```python
from build123d import *

# Parameters (mm, degrees)
SKETCH1_W                        = 56.14
SKETCH1_H                        = 20
BOSS_EXTRUDE1_DEPTH              = 2.49
M3_CLEARANCE_HOLE1_D             = 3.4
M3_CLEARANCE_HOLE1_DEPTH         = 19
M3_CLEARANCE_HOLE1_TIP           = 1.021463052
SKETCH4_W                        = 41.03
SKETCH4_H                        = 20
BOSS_EXTRUDE2_DEPTH              = 8.58
SKETCH5_R                        = 2.98
SKETCH5_R_2                      = 0.928997072
BOSS_EXTRUDE3_DEPTH              = 3.75
SKETCH6_W                        = 8
SKETCH6_H                        = 20
BOSS_EXTRUDE4_DEPTH              = 20
BOSS_EXTRUDE4_2_DEPTH            = 20
SKETCH7_W                        = 41.03
SKETCH7_H                        = 20
BOSS_EXTRUDE5_DEPTH              = 20
SKETCH8_W                        = 56.14
SKETCH8_H                        = 20
BOSS_EXTRUDE6_DEPTH              = 2.46
SKETCH12_W                       = 1.7
SKETCH12_H                       = 24.95
M3_CLEARANCE_HOLE2_AT_2_COUNT    = 2
M3_CLEARANCE_HOLE2_AT_2_PITCH    = 10
M3_CLEARANCE_HOLE2_AT_3_COUNT    = 2
M3_CLEARANCE_HOLE2_AT_3_PITCH    = 50
M3_CLEARANCE_HOLE2_AT_4_COUNT    = 2
M3_CLEARANCE_HOLE2_AT_4_PITCH    = 50.990195136
SKETCH13_W                       = 41.03
SKETCH13_H                       = 20
BOSS_EXTRUDE7_DEPTH              = 39
SKETCH14_R                       = 4
SKETCH14_R_2                     = 1.25
BOSS_EXTRUDE8_DEPTH              = 5.37
SKETCH16_W                       = 0.8
SKETCH16_H                       = 20.00005
TAP_DRILL_FOR_M2_TAP1_AT_2_COUNT = 2
TAP_DRILL_FOR_M2_TAP1_AT_2_PITCH = 25.495097568
TAP_DRILL_FOR_M2_TAP1_AT_3_COUNT = 2
TAP_DRILL_FOR_M2_TAP1_AT_3_PITCH = 10
TAP_DRILL_FOR_M2_TAP1_AT_4_COUNT = 2
TAP_DRILL_FOR_M2_TAP1_AT_4_PITCH = 50
TAP_DRILL_FOR_M2_TAP1_AT_5_COUNT = 2
TAP_DRILL_FOR_M2_TAP1_AT_5_PITCH = 50.990195136
CHAMFER1_SIZE                    = 2
SKETCH19_R                       = 6.18
SKETCH19_R_2                     = 4
BOSS_EXTRUDE10_DEPTH             = 2.12
SKETCH21_W                       = 8
SKETCH21_H                       = 7
CUT_EXTRUDE1_DEPTH               = 28
SKETCH22_W                       = 20
SKETCH22_H                       = 20
CUT_EXTRUDE2_DEPTH               = 8.235
SKETCH23_W                       = 20
SKETCH23_H                       = 20
CUT_EXTRUDE3_DEPTH               = 8.235


with BuildPart() as part:
    # Sketch1 → Boss-Extrude1 (new body)
    with BuildSketch(Plane.XY):
        Rectangle(SKETCH1_W, SKETCH1_H)
    extrude(amount=BOSS_EXTRUDE1_DEPTH)

    # M3 Clearance Hole1
    with Locations(Plane.XY.offset(2.49)):
        with Locations((25, 5), (0, 0), (-25, 5), (-25, -5), (25, -5)):
            Hole(M3_CLEARANCE_HOLE1_D / 2, depth=M3_CLEARANCE_HOLE1_DEPTH)
            with Locations((0, 0, -(M3_CLEARANCE_HOLE1_DEPTH + M3_CLEARANCE_HOLE1_TIP / 2))):  # 118° drill point
                Cone(0, M3_CLEARANCE_HOLE1_D / 2, M3_CLEARANCE_HOLE1_TIP, mode=Mode.SUBTRACT)

    # Sketch4 → Boss-Extrude2 (add)
    with BuildSketch(Plane.XY.offset(2.49)):
        Rectangle(SKETCH4_W, SKETCH4_H)
    extrude(amount=BOSS_EXTRUDE2_DEPTH)

    # Sketch5 → Boss-Extrude3 (add)
    with BuildSketch(Plane.XY.offset(11.07)):
        with Locations((8.73, 0)):
            Circle(SKETCH5_R)
        with Locations((8.73, 0)):
            Circle(SKETCH5_R_2, mode=Mode.SUBTRACT)
    extrude(amount=BOSS_EXTRUDE3_DEPTH)

    # Sketch7 → Boss-Extrude5 (add)
    with BuildSketch(Plane(origin=(0, 0, 0), x_dir=(-1, 0, 0), z_dir=(0, 0, -1))):
        Rectangle(SKETCH7_W, SKETCH7_H)
    extrude(amount=BOSS_EXTRUDE5_DEPTH)

    # Sketch8 → Boss-Extrude6 (add)
    with BuildSketch(Plane(origin=(0, 0, -20), x_dir=(-1, 0, 0), z_dir=(0, 0, -1))):
        Rectangle(SKETCH8_W, SKETCH8_H)
    extrude(amount=BOSS_EXTRUDE6_DEPTH)


with BuildPart() as body_2:
    # Sketch6 → Boss-Extrude4 (new body)
    with BuildSketch(Plane(origin=(0, 0, 0), x_dir=(-1, 0, 0), z_dir=(0, 0, -1))):
        with Locations((-24.75, 0)):
            Rectangle(SKETCH6_W, SKETCH6_H)
    extrude(amount=BOSS_EXTRUDE4_DEPTH)


with BuildPart() as body_3:
    # Sketch6 → Boss-Extrude4 2 (new body)
    with BuildSketch(Plane(origin=(0, 0, 0), x_dir=(-1, 0, 0), z_dir=(0, 0, -1))):
        with Locations((24.75, 0)):
            Rectangle(SKETCH6_W, SKETCH6_H)
    extrude(amount=BOSS_EXTRUDE4_2_DEPTH)


with BuildPart() as m3_clearance_hole2_tool:
    # Sketch12 → M3 Clearance Hole2 (revolve)
    with BuildSketch(Plane(origin=(25, 5, 2.49), x_dir=(0, -1, 0), z_dir=(1, 0, 0))):
        with Locations((0.85, 12.475)):
            Rectangle(SKETCH12_W, SKETCH12_H)
    m3_clearance_hole2 = revolve(axis=Axis((25, 5, 8.84), (0, 0, -1)))


with BuildPart() as part_1:
    add(part.part)

    # M3 Clearance Hole2: cut by m3_clearance_hole2_tool
    add(m3_clearance_hole2_tool.part, mode=Mode.SUBTRACT)


with BuildPart() as body_2_1:
    add(body_2.part)

    # M3 Clearance Hole2: cut by m3_clearance_hole2_tool
    add(m3_clearance_hole2_tool.part, mode=Mode.SUBTRACT)


with BuildPart() as m3_clearance_hole2_at_2_tool:
    # M3 Clearance Hole2 at 2: M3 Clearance Hole2 ×2
    with Locations(*[(0, -i * M3_CLEARANCE_HOLE2_AT_2_PITCH, 0) for i in range(1, M3_CLEARANCE_HOLE2_AT_2_COUNT)]):
        add(m3_clearance_hole2)


with BuildPart() as part_2:
    add(part_1.part)

    # M3 Clearance Hole2 at 2: cut by m3_clearance_hole2_at_2_tool
    add(m3_clearance_hole2_at_2_tool.part, mode=Mode.SUBTRACT)


with BuildPart() as body_2_2:
    add(body_2_1.part)

    # M3 Clearance Hole2 at 2: cut by m3_clearance_hole2_at_2_tool
    add(m3_clearance_hole2_at_2_tool.part, mode=Mode.SUBTRACT)


with BuildPart() as m3_clearance_hole2_at_3_tool:
    # M3 Clearance Hole2 at 3: M3 Clearance Hole2 ×2
    with Locations(*[(-i * M3_CLEARANCE_HOLE2_AT_3_PITCH, 0, 0) for i in range(1, M3_CLEARANCE_HOLE2_AT_3_COUNT)]):
        add(m3_clearance_hole2)


with BuildPart() as part_3:
    add(part_2.part)

    # M3 Clearance Hole2 at 3: cut by m3_clearance_hole2_at_3_tool
    add(m3_clearance_hole2_at_3_tool.part, mode=Mode.SUBTRACT)


with BuildPart() as body_3_1:
    add(body_3.part)

    # M3 Clearance Hole2 at 3: cut by m3_clearance_hole2_at_3_tool
    add(m3_clearance_hole2_at_3_tool.part, mode=Mode.SUBTRACT)


with BuildPart() as m3_clearance_hole2_at_4_tool:
    # M3 Clearance Hole2 at 4: M3 Clearance Hole2 ×2
    with Locations(*[Vector(-0.9805806756909201, -0.19611613513818418, 0) * (i * M3_CLEARANCE_HOLE2_AT_4_PITCH) for i in range(1, M3_CLEARANCE_HOLE2_AT_4_COUNT)]):
        add(m3_clearance_hole2)


with BuildPart() as part_4:
    add(part_3.part)

    # M3 Clearance Hole2 at 4: cut by m3_clearance_hole2_at_4_tool
    add(m3_clearance_hole2_at_4_tool.part, mode=Mode.SUBTRACT)

    # Sketch13 → Boss-Extrude7 (add)
    with BuildSketch(Plane.XY.offset(11.07)):
        Rectangle(SKETCH13_W, SKETCH13_H)
    extrude(amount=-BOSS_EXTRUDE7_DEPTH)

    # Sketch14 → Boss-Extrude8 (add)
    with BuildSketch(Plane(origin=(0, 0, -27.93), x_dir=(-1, 0, 0), z_dir=(0, 0, -1))):
        with Locations(Location((-8.73, 0, 0), (0, 0, 180))):
            Circle(SKETCH14_R)
        with Locations(Location((-8.73, 0, 0), (0, 0, 180))):
            Circle(SKETCH14_R_2, mode=Mode.SUBTRACT)
    extrude(amount=BOSS_EXTRUDE8_DEPTH)


with BuildPart() as body_3_2:
    add(body_3_1.part)

    # M3 Clearance Hole2 at 4: cut by m3_clearance_hole2_at_4_tool
    add(m3_clearance_hole2_at_4_tool.part, mode=Mode.SUBTRACT)

    # Sketch16 → Tap Drill for M2 Tap1 (revolve, cut)
    with BuildSketch(Plane(origin=(-25, -10, -5), x_dir=(0, 0, -1), z_dir=(1, 0, 0))):
        with Locations((0.4, 10.000025)):
            Rectangle(SKETCH16_W, SKETCH16_H)
    tap_drill_for_m2_tap1 = revolve(axis=Axis((-25, -16.35, -5), (0, 1, 0)), mode=Mode.SUBTRACT)

    # Tap Drill for M2 Tap1 at 3: Tap Drill for M2 Tap1 ×2
    with Locations(*[(0, 0, -i * TAP_DRILL_FOR_M2_TAP1_AT_3_PITCH) for i in range(1, TAP_DRILL_FOR_M2_TAP1_AT_3_COUNT)]):
        add(tap_drill_for_m2_tap1, mode=Mode.SUBTRACT)


with BuildPart() as part_5:
    add(part_4.part)

    # Tap Drill for M2 Tap1 at 2: Tap Drill for M2 Tap1 ×2
    with Locations(*[Vector(0.9805806756909201, 0, -0.1961161351381842) * (i * TAP_DRILL_FOR_M2_TAP1_AT_2_PITCH) for i in range(1, TAP_DRILL_FOR_M2_TAP1_AT_2_COUNT)]):
        add(tap_drill_for_m2_tap1, mode=Mode.SUBTRACT)

    # Chamfer1
    chamfer1_edges = [part_5.edges().sort_by_distance(p)[0] for p in [
        (-20.515, 0, 11.07),
        (20.515, 0, 11.07),
    ]]
    chamfer(chamfer1_edges, length=CHAMFER1_SIZE)

    # Sketch19 → Boss-Extrude10 (add)
    with BuildSketch(Plane(origin=(0, 0, -27.93), x_dir=(-1, 0, 0), z_dir=(0, 0, -1))):
        with Locations(Location((-8.73, 0, 0), (0, 0, 180))):
            Circle(SKETCH19_R)
        with Locations(Location((-8.73, 0, 0), (0, 0, 180))):
            Circle(SKETCH19_R_2, mode=Mode.SUBTRACT)
    extrude(amount=BOSS_EXTRUDE10_DEPTH)


with BuildPart() as body_2_3:
    add(body_2_2.part)

    # Tap Drill for M2 Tap1 at 4: Tap Drill for M2 Tap1 ×2
    with Locations(*[(i * TAP_DRILL_FOR_M2_TAP1_AT_4_PITCH, 0, 0) for i in range(1, TAP_DRILL_FOR_M2_TAP1_AT_4_COUNT)]):
        add(tap_drill_for_m2_tap1, mode=Mode.SUBTRACT)

    # Tap Drill for M2 Tap1 at 5: Tap Drill for M2 Tap1 ×2
    with Locations(*[Vector(0.9805806756909202, 0, -0.19611613513818407) * (i * TAP_DRILL_FOR_M2_TAP1_AT_5_PITCH) for i in range(1, TAP_DRILL_FOR_M2_TAP1_AT_5_COUNT)]):
        add(tap_drill_for_m2_tap1, mode=Mode.SUBTRACT)


with BuildPart() as cut_extrude1_tool:
    # Sketch21 → Cut-Extrude1 (new body)
    with BuildSketch(Plane(origin=(0, 10, 0), x_dir=(1, 0, 0), z_dir=(0, 1, 0))):
        with Locations((-24.75, 10)):
            Rectangle(SKETCH21_W, SKETCH21_H)
        with Locations((24.75, 10)):
            Rectangle(SKETCH21_W, SKETCH21_H)
    extrude(amount=-CUT_EXTRUDE1_DEPTH)


with BuildPart() as body_2_4:
    add(body_2_3.part)

    # Cut-Extrude1: cut by cut_extrude1_tool
    add(cut_extrude1_tool.part, mode=Mode.SUBTRACT)


with BuildPart() as body_3_3:
    add(body_3_2.part)

    # Cut-Extrude1: cut by cut_extrude1_tool
    add(cut_extrude1_tool.part, mode=Mode.SUBTRACT)


with BuildPart() as cut_extrude1_piece_1:
    # of the separate pieces the step leaves, piece 1, a body of its own (cut_extrude1_pieces)
    add(body_2_4.part.solids().sort_by_distance((20.75, 10, 0))[0])


with BuildPart() as cut_extrude1_piece_2:
    # of the separate pieces the step leaves, piece 2, a body of its own (cut_extrude1_pieces)
    add(body_2_4.part.solids().sort_by_distance((20.75, 10, -13.5))[0])


with BuildPart() as cut_extrude1_piece_1_of_body_3:
    # of the separate pieces the step leaves, piece 1, a body of its own (cut_extrude1_pieces_of_body_3)
    add(body_3_3.part.solids().sort_by_distance((-28.75, 10, 0))[0])


with BuildPart() as cut_extrude1_piece_2_of_body_3:
    # of the separate pieces the step leaves, piece 2, a body of its own (cut_extrude1_pieces_of_body_3)
    add(body_3_3.part.solids().sort_by_distance((-28.75, 10, -13.5))[0])


with BuildPart() as cut_extrude2_tool:
    # Sketch22 → Cut-Extrude2 (new body)
    with BuildSketch(Plane.ZY.offset(28.75)):
        with Locations((-10, 0)):
            Rectangle(SKETCH22_W, SKETCH22_H)
    extrude(amount=-CUT_EXTRUDE2_DEPTH)


with BuildPart() as cut_extrude1_piece_1_of_body_3_1:
    add(cut_extrude1_piece_1_of_body_3.part)

    # Cut-Extrude2: cut by cut_extrude2_tool
    add(cut_extrude2_tool.part, mode=Mode.SUBTRACT)


with BuildPart() as cut_extrude1_piece_2_of_body_3_1:
    add(cut_extrude1_piece_2_of_body_3.part)

    # Cut-Extrude2: cut by cut_extrude2_tool
    add(cut_extrude2_tool.part, mode=Mode.SUBTRACT)


with BuildPart() as cut_extrude3_tool:
    # Sketch23 → Cut-Extrude3 (new body)
    with BuildSketch(Plane(origin=(28.75, 0, 0), x_dir=(0, 0, -1), z_dir=(1, 0, 0))):
        with Locations((10, 0)):
            Rectangle(SKETCH23_W, SKETCH23_H)
    extrude(amount=-CUT_EXTRUDE3_DEPTH)


with BuildPart() as cut_extrude1_piece_1_1:
    add(cut_extrude1_piece_1.part)

    # Cut-Extrude3: cut by cut_extrude3_tool
    add(cut_extrude3_tool.part, mode=Mode.SUBTRACT)


with BuildPart() as cut_extrude1_piece_2_1:
    add(cut_extrude1_piece_2.part)

    # Cut-Extrude3: cut by cut_extrude3_tool
    add(cut_extrude3_tool.part, mode=Mode.SUBTRACT)


solid = part_5.part
```
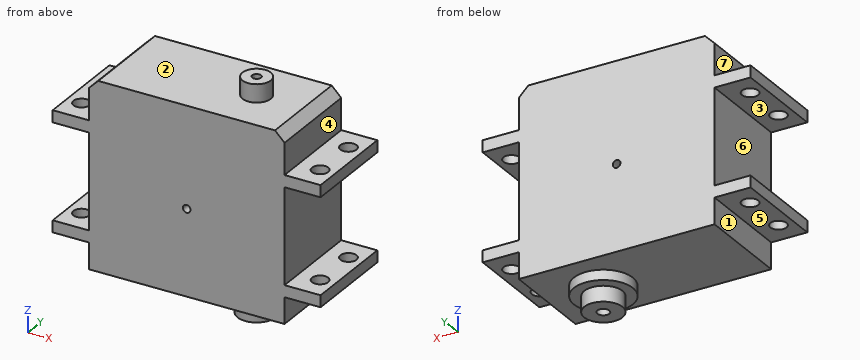
Geometry: final body of the model. Coordinates: model frame, mm. Face numbers are marked on the shaded views. A direction names the side the tool comes from. Give positions to 0.01 mm unless a question says otherwise; leave off trailing zeros. Loops run counter-clockwise (first coordinate to the right, second up) from the corner with the lowest first, then second, coordinate; pieces in that order, holes last. Notation, with made-up numbers: (-35.5, 80.5) -> (4.5, 80.5) arc R6 ccw to (4.5, 89.5) -> close; hole circle Ø2 at (-31.75, 40). An arc over 180 degrees is marked (long way). Use one line per item in the form item = value.
Item 1: Pin query (flat end, axial travel): P1, Ø4, axis at x = 25.5, y = 1, coming from the -Z side; P2, Ø4.5, axis at y = -2, z = -25.5, coming from the -X side (3 decimals); P3, Ø0.9, axis at x = 8.5, y = 0, coming from the +Z side. Return the tip coordinate at first contact, or that it passes through.
A:
P1 = -22.46
P2 = -20.515
P3 = 11.07
Item 2: Line query: probe 1 along X at (y, z) = (5, -21.55); probe 2 along Y at (x, z) = (-25, -21); probe 3 along X at (y, z) = (-1.75, -10) (3 decimals). Output: solid intervals per line, ascending.
A:
probe_1 = -28.07 to -26.7, -23.3 to 23.3, 26.7 to 28.07
probe_2 = -10 to -6.7, -3.3 to 3.3, 6.7 to 10
probe_3 = -20.515 to -0.8, 0.8 to 20.515
Item 3: Section query D-D on x = 8.73. Output: boundary loops of the cut face in (y, z), and give its area (3 significant figures).
A:
outline = (-10, -27.93) -> (-6.18, -27.93) -> (-6.18, -30.05) -> (-4, -30.05) -> (-4, -33.3) -> (-1.25, -33.3) -> (-1.25, -27.93) -> (1.25, -27.93) -> (1.25, -33.3) -> (4, -33.3) -> (4, -30.05) -> (6.18, -30.05) -> (6.18, -27.93) -> (10, -27.93) -> (10, 11.07) -> (2.98, 11.07) -> (2.98, 14.82) -> (0.93, 14.82) -> (0.93, 11.07) -> (-0.93, 11.07) -> (-0.93, 14.82) -> (-2.98, 14.82) -> (-2.98, 11.07) -> (-10, 11.07) -> close
area = 834 mm^2
Item 4: Section query C-C on x = -25. Output: boundary loops of the cut face in (y, z), and give its area (3 significant figures).
A:
outline = (-10, -22.46) -> (-6.7, -22.46) -> (-6.7, -20) -> (-10, -20) -> close; (-10, 0) -> (-6.7, 0) -> (-6.7, 2.49) -> (-10, 2.49) -> close; (-3.3, -22.46) -> (3.3, -22.46) -> (3.3, -20) -> (-3.3, -20) -> close; (-3.3, 0) -> (3.3, 0) -> (3.3, 2.49) -> (-3.3, 2.49) -> close; (6.7, -22.46) -> (10, -22.46) -> (10, -20) -> (6.7, -20) -> close; (6.7, 0) -> (10, 0) -> (10, 2.49) -> (6.7, 2.49) -> close
area = 65.3 mm^2
Item 5: Draft query along Z for the marked faces 1, 2 and 3. Return one class per face: pulls with the +Z half, pulls with the -Z half, needs draft (parallel to the pull), parting line crosses it, or undercut.
A:
face_1 = needs draft
face_2 = pulls with the +Z half
face_3 = undercut
Item 6: Access query for the marked faces 4, 5, 6 and 7. Directions: +Z, -Z, +X, -X, +Y, -Y. A direction counts if a zero-diameter tool reaches every point of the face in a straight line with its end or side. Return the directions, or none.
A:
face_4 = +Z, +X, +Y, -Y
face_5 = -Z, -X, +Y, -Y
face_6 = -X, +Y, -Y
face_7 = +Z, -X, +Y, -Y
Item 7: Section query A-A on z = -10. Output: boundary loops of the cut face in (x, y) (3 decimals), and give its area (3 significant figures).
A:
outline = (-20.515, -10) -> (-0.8, -10) -> (-0.8, 10) -> (-20.515, 10) -> close; (0.8, -10) -> (20.515, -10) -> (20.515, 10) -> (0.8, 10) -> close
area = 789 mm^2
Item 8: Section query B-B on y = -8. Output: boundary loops of the cut face in (x, z) (3 decimals), and give its area (3 significant figures).
A:
outline = (-28.07, -22.46) -> (-20.515, -22.46) -> (-20.515, -27.93) -> (20.515, -27.93) -> (20.515, -22.46) -> (28.07, -22.46) -> (28.07, -20) -> (20.515, -20) -> (20.515, 0) -> (28.07, 0) -> (28.07, 2.49) -> (20.515, 2.49) -> (20.515, 9.07) -> (18.515, 11.07) -> (-18.515, 11.07) -> (-20.515, 9.07) -> (-20.515, 2.49) -> (-28.07, 2.49) -> (-28.07, 0) -> (-20.515, 0) -> (-20.515, -20) -> (-28.07, -20) -> close; hole circle Ø1.6 at (0, -10)
area = 1,670 mm^2
